Read the model definition and answer for the solid it produces. Units are mm, in the model's axes. A direction names the side the tool comes from. Give positions to 0.01 mm unless a question says otherwise; leave off trailing zeros. Loops run counter-clockwise (first coordinate to the right, second up) from the corner with the lowest first, then second, coordinate; pieces in that order, holes last. Notation, with made-up numbers: (87, -8.75) - (118, -8.75) arc R13 cw to (118, 3.25) - close; hole circle Ø6 at (77, 82.25). An arc over 180 degrees is marked (long way). Use a Markdown table: item, result. Add a question column.
Item 1: A cutting plane is placed at D-D (z = 19.5). Determine the outline of the cut face in (x, y), plus the area to 3 significant figures.
Item 2: A cutting plane is placed at A-A (y = 8.5). Determine the outline of the cut face in (x, z).
Item 3: Each of these flat-tipped pins is pushed along its axis until it touches: P1, Ø10, axis at x = -14.5, y = 16, coming from the -Z side; P2, Ø6, axis at y = 12, z = 19, coming from the -X side; P3, Ø2, axis at y = 17, z = 30, coming from the +X side. Where does it stop, or does it pass through?
Item 4: Consider probe 1 along Z at (x, y) = (0.75, 6.25); probe 2 along Y at (x, z) = (-16, 41.5); probe 3 along X at (y, z) = (13.25, 3.5). Determine where each line is inside the solid, lowest interval first. Write a range as [from, to].
Item 5: A cutting plane is placed at C-C (z = 9.5). Determine the outline of the cut face in (x, y), plus the area to 3 significant figures.
Item 6: Which of the six approach directions +Z, -Z, +X, -X, +Y, -Y give full straight-line access (tool end or side, diameter ignored) to faces 1 (the face through (0.4, 11.1, 25)), 2 (the face through (0, 8, 12)), 3 (the face through (1, 9, 0))?
Item 7: A cutting plane is placed at B-B (z = 32). Determine the outline of the cut face in (x, y).
from build123d import *

# Parameters (mm, degrees)
EXTRUDE_THIN1_DEPTH = 70
CUT_EXTRUDE1_DEPTH  = 19
CUT_EXTRUDE2_DEPTH  = 19
FILLET1_R           = 2


with BuildPart() as part:
    # Sketch1 → Extrude-Thin1 (new body)
    with BuildSketch(Plane.XY):
        Polygon((0, 0), (0, 16), (-20, 16), (-20, 18), (2, 18), (2, 0), align=None)
    extrude(amount=EXTRUDE_THIN1_DEPTH)

    # Sketch2 → Cut-Extrude1 (cut, through all)
    with BuildSketch(Plane(origin=(0, 18, 0), x_dir=(1, 0, 0), z_dir=(0, 1, 0))):
        Polygon((2, -25), (-5.822, -25), (-5.822, -33), (-18, -70), (2, -70), align=None)
    extrude(amount=-CUT_EXTRUDE1_DEPTH, mode=Mode.SUBTRACT)

    # Sketch3 → Cut-Extrude2 (cut, through all)
    with BuildSketch(Plane(origin=(0, 18, 0), x_dir=(1, 0, 0), z_dir=(0, 1, 0))):
        Polygon((-20, -23.835071852), (0, 0), (-20, 0), align=None)
    extrude(amount=-CUT_EXTRUDE2_DEPTH, mode=Mode.SUBTRACT)

    # Fillet1
    fillet1_edges = [part.edges().sort_by_distance(p)[0] for p in [
        (-18, 17, 70),
        (-5.822, 17, 33),
        (-5.822, 17, 25),
        (-20, 17, 23.835071852),
    ]]
    fillet(fillet1_edges, radius=FILLET1_R)


solid = part.part
Geometry says:
| question | item | result |
|---|---|---|
| 1 | outline | (-16.36, 16) - (0, 16) - (0, 0) - (2, 0) - (2, 18) - (-16.36, 18) - close |
| 1 | area | 68.7 mm² |
| 2 | outline | (0, 0) - (2, 0) - (2, 25) - (0, 25) - close |
| 3 | P1 | z = 11.32 |
| 3 | P2 | x = 0 |
| 3 | P3 | x = -5.82 |
| 4 | probe 1 | [0, 25] |
| 4 | probe 2 | [16, 18] |
| 4 | probe 3 | [0, 2] |
| 5 | outline | (-7.97, 16) - (0, 16) - (0, 0) - (2, 0) - (2, 18) - (-7.97, 18) - close |
| 5 | area | 51.9 mm² |
| 6 | face 1 | +Z, +X, +Y, -Y |
| 6 | face 2 | +Z, -Z, -X, -Y |
| 6 | face 3 | -Z, +X, -X, +Y, -Y |
| 7 | outline | (-20, 16) - (-5.82, 16) - (-5.82, 18) - (-20, 18) - close |
